```python
from build123d import *

# Parameters (mm, degrees)
BOSS_EXTRUDE1_DEPTH     = 12.7
SKETCH2_R               = 3.175
CUT_EXTRUDE1_DEPTH      = 13.7
SKETCH3_W               = 6.35
SKETCH3_H               = 11.43
CUT_EXTRUDE2_DEPTH      = 86.600261098
SKETCH4_R               = 4
CUT_EXTRUDE3_DEPTH      = 13.7
F_1_4_CLEARANCE_HOLE1_D = 6.7564


with BuildPart() as part:
    # Sketch1 → Boss-Extrude1 (new body)
    with BuildSketch(Plane.XY):
        Polygon((-42.800130549, -5.715), (-10.39539802, -41.91), (10.39539802, -41.91), (42.800130549, -5.715), (42.800130549, 5.715), (-42.800130549, 5.715), align=None)
    extrude(amount=-BOSS_EXTRUDE1_DEPTH)

    # Sketch2 → Cut-Extrude1 (cut, through all)
    with BuildSketch(Plane.XY):
        Circle(SKETCH2_R)
    extrude(amount=-CUT_EXTRUDE1_DEPTH, mode=Mode.SUBTRACT)

    # Sketch3 → Cut-Extrude2 (cut, through all)
    with BuildSketch(Plane(origin=(42.800130549, 0, 0), x_dir=(0, 0, -1), z_dir=(1, 0, 0))):
        with Locations((9.525, 0)):
            Rectangle(SKETCH3_W, SKETCH3_H)
    extrude(amount=-CUT_EXTRUDE2_DEPTH, mode=Mode.SUBTRACT)

    # Sketch4 → Cut-Extrude3 (cut, through all)
    with BuildSketch(Plane.XY):
        with Locations((0, -15.24)):
            Circle(SKETCH4_R)
    extrude(amount=-CUT_EXTRUDE3_DEPTH, mode=Mode.SUBTRACT)

    # 1/4 Clearance Hole1 (through all)
    with Locations(Plane(origin=(0, 0, -6.35), x_dir=(-1, 0, 0), z_dir=(0, 0, -1))):
        with Locations((-37.720130549, 0), (37.720130549, 0)):
            Hole(F_1_4_CLEARANCE_HOLE1_D / 2)


solid = part.part
```
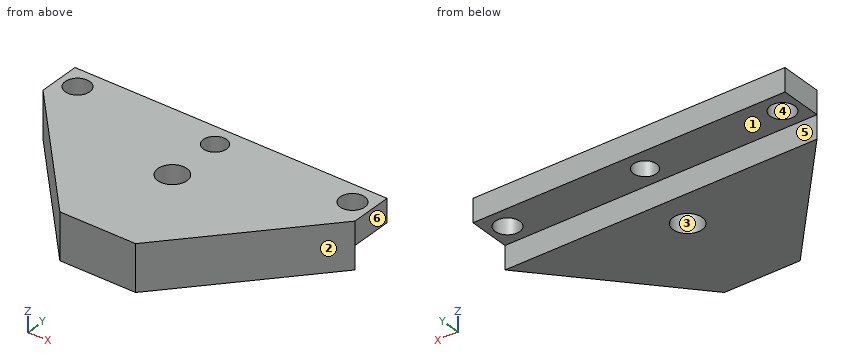
Build history of the part. All positions in model axes, mm. Face numbers are marked on the shaded views. A direction names the side the tool comes from. Give positions to 0.01 mm unless a question says otherwise; leave off trailing zeros. Order: outer loops, then holes, each group sorted by start corner. A loop starts at its lowest first (then second) coordinate and runs counter-clockwise, first axis right, second up. Notation, with made-up numbers: M 36,-4.75 L 82,-4.75 A22 ccw 82,11.25 Z; hole C -7.75,0.5 d9. An arc over 180 degrees is marked long. Return JSON: item names as keys, results as strings.
Q1. Band-saw the part on C-C (y = -15.24). Give the cut face in (x, z).
Answer list:
{"outline": "M -34.27,-12.7 L -4,-12.7 L -4,0 L -34.27,0 Z; M 4,-12.7 L 34.27,-12.7 L 34.27,0 L 4,0 Z"}
Q2. Two-plate mould, pull along Y, no slides. Class the marked faces 3, 4, 5 and 6: pulls with the +Y half, pulls with the -Y half, needs draft (parallel to the pull), parting line crosses it, or undercut.
Answer list:
{"face 3": "undercut", "face 4": "undercut", "face 5": "pulls with the +Y half", "face 6": "needs draft"}
Q3. Wall check: probe 1 along Y at (x, z) = (0, -2.5) (3 decimals); probe 2 along X at (y, z) = (1.5, -4.75); probe 3 along Y at (x, z) = (0, -6.5) (3 decimals). Give the ranges that are in metal, low to high. Write a range as from..to.
Answer list:
{"probe 1": "y = -41.91..-19.24, -11.24..-3.175, 3.175..5.715", "probe 2": "x = -42.8..-40.75, -34.69..-2.8, 2.8..34.69, 40.75..42.8", "probe 3": "y = -41.91..-19.24, -11.24..-5.715"}
Q4. Flat gauge pins, fed straight in: pin 1 (2 mm diameter, centred on y = -20, z = -10.5, fed in from -X); pin 2 (2 mm diameter, centred on y = -35.5, z = -2, fed in from -X). Where does each tip first touch, or does it go through?
Answer list:
{"pin 1": "stops at x = -30.91", "pin 2": "stops at x = -17.03"}
Q5. Band-saw the part on A-A (y = 0). Give the cut face in (x, z) (3 decimals), then the cut area to 3 significant figures.
Answer list:
{"outline": "M -42.8,-6.35 L -41.098,-6.35 L -41.098,0 L -42.8,0 Z; M -34.342,-6.35 L -3.175,-6.35 L -3.175,0 L -34.342,0 Z; M 3.175,-6.35 L 34.342,-6.35 L 34.342,0 L 3.175,0 Z; M 41.098,-6.35 L 42.8,-6.35 L 42.8,0 L 41.098,0 Z", "area": "417 mm^2"}
Q6. 3-axis set-ups, long thin cutter, end or side, ignore diameter. For the marked faces 1 and 2: which of +Z, -Z, +X, -X, +Y, -Y reach the whole face in a straight line?
Answer list:
{"face 1": "-Z, +X, -X, +Y", "face 2": "+Z, -Z, +X, -Y"}
Q7. Band-saw the part on B-B (x = 0). Give the cut face in (y, z) (3 decimals).
Answer list:
{"outline": "M -41.91,-12.7 L -19.24,-12.7 L -19.24,0 L -41.91,0 Z; M -11.24,-12.7 L -5.715,-12.7 L -5.715,-6.35 L -3.175,-6.35 L -3.175,0 L -11.24,0 Z; M 3.175,-6.35 L 5.715,-6.35 L 5.715,0 L 3.175,0 Z"}
Q8. Band-saw the part on D-D (z = -10.25). Give the cut face in (x, y) (3 decimals).
Answer list:
{"outline": "M -42.8,-5.715 L -10.395,-41.91 L 10.395,-41.91 L 42.8,-5.715 Z; hole C 0,-15.24 d8"}
